Check sheet for the modelled part. Datum: model origin and axes. Units: mm. A direction names the side the tool comes from. Round coordinates to 2 decimals unless told otherwise and drop trailing zeros. Write each loop counter-clockwise with the first axis right and the second up, starting at its lowest first coordinate (ties: lowest second). Pieces come first, ordered by that corner, then holes. Notation, with made-up numbers: M -10,65.5 L 25,65.5 A11 cw 25,74.5 Z; hole C 22,4 d3. An arc over 180 degrees is marked long. Put each result on its own line as item: value.
```python
from build123d import *

# Parameters (mm, degrees)
BOSS_EXTRUDE1_DEPTH                      = 15
FILLET1_R                                = 60
SKETCH_2_R                               = 25
CUT_EXTRUDE_2_DEPTH                      = 16
CUT_EXTRUDE_START                        = -10
SKETCH_1_W                               = 60
SKETCH_1_H                               = 60
CUT_EXTRUDE_1_DEPTH                      = 10
SKETCH_3_W                               = 40
SKETCH_3_H                               = 33
CUT_EXTRUDE_3_DEPTH                      = 7
M7X1_0_1_D                               = 6
M7X1_0_1_DEPTH                           = 17
M7X1_0_1_TIP                             = 1.802581857
PATTERN_CIRCULAR_1_COUNT                 = 6
SKETCH5_R                                = 13
CUT_EXTRUDE2_DEPTH                       = 16
CUT_EXTRUDE1_START                       = -15
SKETCH4_W                                = 42
SKETCH4_H                                = 42
CUT_EXTRUDE1_DEPTH                       = 8
CUT_EXTRUDE3_START                       = -15
CUT_EXTRUDE3_DEPTH                       = 8
FILLET2_R                                = 3
CHAMFER1_SIZE                            = 1
CBORE_FOR_M3_PAN_HEAD_SCREW1_D           = 3.4
CBORE_FOR_M3_PAN_HEAD_SCREW1_CBORE_D     = 7
CBORE_FOR_M3_PAN_HEAD_SCREW1_CBORE_DEPTH = 2.4
FILLET6_R                                = 4


with BuildPart() as part:
    # Sketch2 → Boss-Extrude1 (new body)
    with BuildSketch(Plane.XY):
        with BuildLine():
            Line((-6.167694754, -49.941502997), (339.564451041, -49.941502997))
            ThreePointArc((339.564451041, -49.941502997), (456.832305246, -17.941502997), (339.564451041, 14.058497003))
            Line((339.564451041, 14.058497003), (-6.167694754, 14.058497003))
            ThreePointArc((-6.167694754, 14.058497003), (-38.167694754, -17.941502997), (-6.167694754, -49.941502997))
        make_face()
    extrude(amount=BOSS_EXTRUDE1_DEPTH)

    # Fillet1
    fillet1_edges = [part.edges().sort_by_distance(p)[0] for p in [
        (339.564451041, 14.058497003, 7.5),
        (339.564451041, -49.941502997, 7.5),
    ]]
    fillet(fillet1_edges, radius=FILLET1_R)

    # 草圖2 → 除料-伸長2 (cut, through all)
    with BuildSketch(Plane(origin=(0, 0, 0), x_dir=(-1, 0, 0), z_dir=(0, 0, -1))):
        with Locations((-393.832305246, -17.941502997)):
            Circle(SKETCH_2_R)
    extrude(amount=-CUT_EXTRUDE_2_DEPTH, mode=Mode.SUBTRACT)

    # 草圖1 → 除料-伸長1 (cut)
    with BuildSketch(Plane(origin=(0, 0, 0), x_dir=(-1, 0, 0), z_dir=(0, 0, -1)).offset(CUT_EXTRUDE_START)):
        with Locations((-393.832305246, -17.941502997)):
            Rectangle(SKETCH_1_W, SKETCH_1_H)
    extrude(amount=CUT_EXTRUDE_1_DEPTH, mode=Mode.SUBTRACT)

    # 草圖3 → 除料-伸長3 (cut)
    with BuildSketch(Plane(origin=(0, 0, 0), x_dir=(-1, 0, 0), z_dir=(0, 0, -1))):
        with Locations((-393.832305246, -64.441502997)):
            Rectangle(SKETCH_3_W, SKETCH_3_H)
    extrude(amount=-CUT_EXTRUDE_3_DEPTH, mode=Mode.SUBTRACT)

    # M7x1.0 螺紋孔1
    with Locations(Plane(origin=(0, 0, 10), x_dir=(-1, 0, 0), z_dir=(0, 0, -1))):
        with Locations((-368.832305246, 7.058497003), (-368.832305246, -42.941502997), (-418.832305246, -42.941502997), (-418.832305246, 7.058497003)):
            Hole(M7X1_0_1_D / 2, depth=M7X1_0_1_DEPTH)
            with Locations((0, 0, -(M7X1_0_1_DEPTH + M7X1_0_1_TIP / 2))):  # 118° drill point
                Cone(0, M7X1_0_1_D / 2, M7X1_0_1_TIP, mode=Mode.SUBTRACT)

    # 草圖8 → M8x1.25 螺紋孔1 (revolve, cut)
    with BuildSketch(Plane(origin=(448.332305246, -17.941502997, 15), x_dir=(0, -1, 0), z_dir=(1, 0, 0))):
        Polygon((0, 0), (0, 21.792926105), (3.4, 19.75), (3.4, 0), align=None)
    m8x1_25_1 = revolve(axis=Axis((448.332305246, -17.941502997, 21.35), (0, 0, -1)), mode=Mode.SUBTRACT)

    # 環狀複製排列1: M8x1.25 螺紋孔1 ×6 about axis
    pattern_circular_1_axis = Axis((393.832305246, -17.941502997, 0), (0, 0, 1))
    for i in range(1, PATTERN_CIRCULAR_1_COUNT):
        add(m8x1_25_1.rotate(pattern_circular_1_axis, i * 360 / PATTERN_CIRCULAR_1_COUNT), mode=Mode.SUBTRACT)

    # Sketch5 → Cut-Extrude2 (cut, through all)
    with BuildSketch(Plane.XY.offset(15)):
        with Locations((-6.167694754, -17.941502997)):
            Circle(SKETCH5_R)
    extrude(amount=-CUT_EXTRUDE2_DEPTH, mode=Mode.SUBTRACT)

    # Sketch4 → Cut-Extrude1 (cut)
    with BuildSketch(Plane.XY.offset(15).offset(CUT_EXTRUDE1_START)):
        with Locations((-6.167694754, -17.941502997)):
            Rectangle(SKETCH4_W, SKETCH4_H)
    extrude(amount=CUT_EXTRUDE1_DEPTH, mode=Mode.SUBTRACT)

    # Sketch8 → Cut-Extrude3 (cut)
    with BuildSketch(Plane.XY.offset(15).offset(CUT_EXTRUDE3_START)):
        with BuildLine():
            Line((-19.554255179, 3.058497003), (7.21886567, 3.058497003))
            ThreePointArc((7.21886567, 3.058497003), (-6.167694754, 11.058497003), (-19.554255179, 3.058497003))
        make_face()
    extrude(amount=CUT_EXTRUDE3_DEPTH, mode=Mode.SUBTRACT)

    # Fillet2
    fillet2_edges = [part.edges().sort_by_distance(p)[0] for p in [
        (-27.167694754, 3.058497003, 4),
        (-27.167694754, -38.941502997, 4),
        (14.832305246, -38.941502997, 4),
        (14.832305246, 3.058497003, 4),
        (7.21886567, 3.058497003, 4),
        (-19.554255179, 3.058497003, 4),
    ]]
    fillet(fillet2_edges, radius=FILLET2_R)

    # Chamfer1
    chamfer1_edges = [part.edges().sort_by_distance(p)[0] for p in [
        (153.012579622, 14.058497003, 0),
        (153.012579622, 14.058497003, 15),
        (362.287186837, -72.475029424, 0),
        (456.832305246, -17.941502997, 15),
        (333.492115408, 17.966238505, 0),
        (333.492115408, 17.966238505, 15),
        (333.492115408, -53.849244499, 0),
        (333.492115408, -53.849244499, 15),
        (-38.167694754, -17.941502997, 15),
        (448.365831673, 13.603615412, 0),
        (153.012579622, -49.941502997, 0),
        (-38.167694754, -17.941502997, 0),
        (153.012579622, -49.941502997, 15),
    ]]
    chamfer(chamfer1_edges, length=CHAMFER1_SIZE)

    # CBORE for M3 Pan Head Screw1 (through all)
    with Locations(Plane(origin=(0, 0, 15), x_dir=(-1, 0, 0), z_dir=(0, 0, 1))):
        with Locations((21.667694754, 2.441502997), (21.653333262, 33.427141505), (-9.317943754, 33.427141505), (-9.332305246, 2.441502997)):
            CounterBoreHole(CBORE_FOR_M3_PAN_HEAD_SCREW1_D / 2, CBORE_FOR_M3_PAN_HEAD_SCREW1_CBORE_D / 2, CBORE_FOR_M3_PAN_HEAD_SCREW1_CBORE_DEPTH)

    # Fillet6
    fillet6_edges = [part.edges().sort_by_distance(p)[0] for p in [
        (363.832305246, -47.941502997, 5),
        (363.832305246, 12.058497003, 5),
        (423.832305246, 12.058497003, 5),
        (423.832305246, -47.941502997, 5),
    ]]
    fillet(fillet6_edges, radius=FILLET6_R)


solid = part.part
```
1. Cross-section at A-A (x = 140). Enter the section's corners in (y, z).
Computed values:
outline: M -49.94,1 L -48.94,0 L 13.06,0 L 14.06,1 L 14.06,14 L 13.06,15 L -48.94,15 L -49.94,14 Z
2. Cross-section at B-B (z = 3.75). Count the separate pieces of the cut face and the enclosed holes in it, then the cut area to 3 significant figures.
Computed values:
separate pieces: 1
enclosed holes: 7
area: 29,000 mm2
3. Scan lines: probe 1 along X at (y, z) = (31.5, 4); probe 2 along X at (y, z) = (-20.5, 10.25); probe 3 along X at (y, z) = (6, 3.5). Record each from-to range of solid material in increasing order.
Computed values:
probe 1: x = 354.79 to 364.03, 369.14 to 418.53, 423.64 to 432.88
probe 2: x = -38.07 to -18.91, 6.58 to 337.09, 341.57 to 368.96, 418.7 to 446.09, 450.57 to 456.78
probe 3: x = -27.4 to -17.49, 5.15 to 363.83, 423.83 to 452.11
4. Depth check by flat-ended pin: pin 1 Ø7.5 at (y, z) = (-58, 5) entering from +X; pin 2 Ø5 at (y, z) = (-0.5, 10.5) entering from +X; pin 3 Ø6 at (y, z) = (-11.5, 9.5) entering from -X. Enter the tip coordinate at first touch or a pass-through.
Computed values:
pin 1: stops at x = 445.32
pin 2: stops at x = 455.03
pin 3: stops at x = -37.98
5. Access from +Z, -Z, +X, -X, +Y, -Y to the whole of each face (thin tool, end or side, straight path). Record for faces 4 (the flat face through (394, -64, 7)), 5 (the flat face through (155, 14.058, 7)), 6 (the cylindrical face through (333.207, -53.742, 7.591)), 7 (the cylindrical face through (-5.96, 11.057, 3.944)).
Computed values:
face 4: -Z, -Y
face 5: +Z, -Z, -X, +Y
face 6: +Z, -Z, -X, -Y
face 7: -Z
6. Release check for a two-part mould opening along X. For faces 1 (the flat face through (-27.168, -18, 4)), 2 (the flat face through (151, -49.942, 7)), 3 (the conical face through (-37.32, -17.26, 14.84)) record: +X half, -X half, draft (parallel to the pull), parting line (faces both ways), or undercut.
Computed values:
face 1: undercut
face 2: draft
face 3: -X half
